Could you check a few things on this model? Use its own coordinates, in mm. A direction names the side the tool comes from. Give positions to 0.01 mm unless a question says otherwise; leave off trailing zeros. Loops run counter-clockwise (first coordinate to the right, second up) from the corner with the lowest first, then second, coordinate; pieces in that order, holes last. Notation, with made-up numbers: M 24,-7.5 L 53,-7.5 A21 ccw 53,3.5 Z; hole C 59.25,-6 d7. An arc over 180 degrees is marked long. Answer in a Markdown table with one row per item. Add a question column.
1. I'm going to push flat-ended pins straight in: pin 1 Ø3 at (x, z) = (84.8, -39.5) entering from -Y; pin 2 Ø3.5 at (y, z) = (1, -13) entering from -X; pin 3 Ø1.5 at (y, z) = (1, -22) entering from +X. Where does each tip first touch, or does it pass through?
2. If we section it at A-A on x = 108: List the corners of the cut face in (y, z) for me, then the cut area to 4 significant figures.
3. If we section it at B-B on z = -8: Count the separate pieces of the cut face and the enclosed holes in it, then the cut area to 3 significant figures.
4. Which directions (+Z, -Z, +X, -X, +Y, -Y) give clear straight access to the entire face, cutting with the end or side of a thin tool? Please do faces 4 (the flat face through (45, 9, -2.9)), 5 (the flat face through (12, 3, -23)), 6 (the flat face through (51.9, 9, -1)), 7 (the flat face through (37, 4, -39)), 8 (the flat face through (120, 4, -23)).
5. If we section it at D-D on z = -22: List the corners of the cut face in (x, y) for me.
6. Thinking about a two-plate mould opening in X: for faces 1 (the cylindrical face through (36.567, 6.958, -39.803)), 2 (the flat face through (108, 3, -23)), 3 (the flat face through (96, 1, -23)), which applies, released by +X, released by -X, zero draft, split by the parting line, or undercut?
7. If we section it at C-C on x = 72.5: List the corners of the cut face in (y, z) for me, then the cut area to 3 significant figures.
8. I need wall thicknesses on line 1 along Z through (x, y) = (108, 3.95); line 2 along X through (y, z) = (4.9, -8); line 3 along Z through (x, y) = (77, 8.75). Which ranges of each line are inside material? Lowest first, please. Write a range as from..to.
Autodesk Inventor part; units mm, degrees
ref_plane "YZ Plane" through (0, 0, 0) normal (1, 0, 0) x (0, 1, 0)
ref_plane "XZ Plane" through (0, 0, 0) normal (0, 1, 0) x (-1, 0, 0)
ref_plane "XY Plane" through (0, 0, 0) normal (0, 0, 1) x (1, 0, 0)
sketch "スケッチ1" plane through (0, 0, 0) normal (0, 1, 0) x (-1, 0, 0)
  line L0 (0, 0) -> (-120, 0)
  line L1 (-120, 0) -> (-120, -47.5)
  line L2 (-120, -47.5) -> (0, -47.5)
  line L3 (0, -47.5) -> (0, 0)
  dimension "d0" = 120
  dimension "d1" = 47.5
extrude "押し出し1" add sketch "スケッチ1" along normal blind 6
ref_plane "作業平面1" through (0, 0, 0) normal (0, 0, 1) x (1, 0, 0)
ref_plane "作業平面2" through (0, 6, 0) normal (0, 1, 0) x (1, 0, 0)
sketch "スケッチ3" plane through (0, 6, 0) normal (0, 1, 0) x (1, 0, 0)
  line L0 (120, 47.5) -> (0, 47.5)
  line L1 (0, 0) -> (120, 0)
  line L2 (30, 47.5) -> (90, 47.5)
  line L3 (90, 47.5) -> (90, 0)
  line L4 (90, 0) -> (30, 0)
  line L5 (30, 0) -> (30, 47.5)
  point P0 (30, 0)
  point P1 (60, 47.5)
  point P2 (60, 47.5)
  point P3 (60, 47.5)
  dimension "d9" = 60
  dimension "d50" = 0
extrude "押し出し3" add sketch "スケッチ3" along normal blind 4
ref_plane "作業平面3" through (0, 10, 0) normal (0, 1, 0) x (1, 0, 0)
sketch "スケッチ4" plane through (0, 10, 0) normal (0, 1, 0) x (1, 0, 0)
  line L0 (38.7, 45.5) -> (81.3, 45.5)
  line L1 (81.3, 45.5) -> (81.3, 2.9)
  line L2 (81.3, 2.9) -> (38.7, 2.9)
  line L3 (38.7, 2.9) -> (38.7, 45.5)
  line L4 (90, 47.5) -> (30, 47.5)
  line L5 (90, 0) -> (90, 47.5)
  point P0 (0, 0)
  point P1 (90, 23.75)
  point P2 (60, 47.5)
  dimension "d14" = 42.6
  dimension "d15" = 42.6
extrude "押し出し4" cut sketch "スケッチ4" against normal blind 2
sketch "スケッチ5" plane through (120, 0, 0) normal (0, 0, 1) x (1, 0, 0)
  line L0 (-30, 10) -> (-90, 10)
  line L1 (-38.7, 8) -> (-81.3, 8)
  line L2 (-68.1, 10) -> (-51.9, 10)
  line L3 (-51.9, 10) -> (-51.9, 8)
  line L4 (-51.9, 8) -> (-68.1, 8)
  line L5 (-68.1, 8) -> (-68.1, 10)
  point P0 (-120, 0)
  dimension "d20" = 16.2
extrude "押し出し5" cut sketch "スケッチ5" against normal blind 3
sketch "スケッチ6" plane through (0, 10, 0) normal (0, 1, 0) x (1, 0, 0)
  line L0 (90, 47.5) -> (30, 47.5)
  line L1 (144, 0) -> (-24, 0)
  line L2 (30, 47.5) -> (30, 0)
  line L3 (90, 0) -> (90, 47.5)
  line L4 (38.7, 2.9) -> (38.7, 45.5)
  point P0 (0, 0)
  point P1 (35.2, 39.5)
  point P2 (35.2, 8)
  point P3 (84.8, 8)
  point P4 (84.8, 39.5)
  dimension "d27" = 8
  dimension "d28" = 8
  dimension "d29" = 8
  dimension "d30" = 8
  dimension "d31" = 5.2
  dimension "d32" = 5.2
  dimension "d33" = 5.2
  dimension "d34" = 5.2
  dimension "d49" = 49.6
  dimension "d75" = 3.5
hole "穴1" at (35.2, 10, -39.5) at (35.2, 10, -8) at (84.8, 10, -8) at (84.8, 10, -39.5) direction (0, -1, 0) diameter 2.8 end through all
sketch "スケッチ7" plane through (0, 0, 0) normal (0, -1, 0) x (1, 0, 0)
  circle A0 centre (35.2, -8) radius 1.4
  circle A1 centre (35.2, -8) radius 3.5
  circle A2 centre (84.8, -8) radius 1.4
  circle A3 centre (84.8, -8) radius 3.5
  circle A4 centre (84.8, -39.5) radius 1.4
  circle A5 centre (84.8, -39.5) radius 3.5
  circle A6 centre (35.2, -39.5) radius 1.4
  circle A7 centre (35.2, -39.5) radius 3.5
  point P0 (0, 0)
  dimension "d42" = 7
  dimension "d43" = 7
  dimension "d44" = 7
  dimension "d45" = 7
extrude "押し出し6" cut sketch "スケッチ7" against normal blind 4 contours A0 | A1 | A3 | A4 | A5 | A6 | A7
ref_plane "作業平面4" through (0, 0, 0) normal (0, -1, 0) x (1, 0, 0)
sketch "スケッチ8" plane through (0, 0, 0) normal (0, -1, 0) x (1, 0, 0)
  line L0 (0, 0) -> (24, 0)
  line L1 (24, 0) -> (24, -47.5)
  line L2 (24, -47.5) -> (0, -47.5)
  line L3 (0, -47.5) -> (0, 0)
  line L4 (120, 0) -> (120, -47.5)
  line L5 (120, 0) -> (96, 0)
  line L6 (96, 0) -> (96, -47.5)
  line L7 (96, -47.5) -> (120, -47.5)
  line L8 (120, -47.5) -> (120, 0)
  dimension "d53" = 24
  dimension "d54" = 47.5
  dimension "d55" = 24
  dimension "d56" = 47.5
extrude "押し出し7" cut sketch "スケッチ8" against normal blind 3
ref_plane "作業平面5" through (0, 3, 0) normal (0, -1, 0) x (1, 0, 0)
sketch "スケッチ9" plane through (0, 3, 0) normal (0, -1, 0) x (1, 0, 0)
  line L0 (0, -47.5) -> (0, 0)
  line L1 (0, 0) -> (24, 0)
  line L2 (24, -47.5) -> (0, -47.5)
  line L3 (120, 0) -> (120, -47.5)
  line L4 (96, 0) -> (120, 0)
  line L5 (120, -47.5) -> (96, -47.5)
  line L6 (24, 0) -> (24, -47.5)
  point P0 (12, -8)
  point P1 (12, -39.5)
  point P2 (108, -8)
  point P3 (108, -39.5)
  point P4 (12, 0)
  dimension "d60" = 12
  dimension "d61" = 8
  dimension "d62" = 8
  dimension "d63" = 12
  dimension "d64" = 12
  dimension "d65" = 12
  dimension "d66" = 8
  dimension "d67" = 8
  dimension "d76" = 12
hole "穴2" at (12, 3, -8) at (12, 3, -39.5) at (108, 3, -8) at (108, 3, -39.5) direction (0, 1, 0) diameter 6 end through all
properties part number "motor_mount1_3D プリント"
Results:
| question | item | result |
|---|---|---|
| 1 | pin 1 | y = 4 |
| 1 | pin 2 | x = 24 |
| 1 | pin 3 | x = 96 |
| 2 | outline | M 3,-47.5 L 6,-47.5 L 6,-42.5 L 3,-42.5 Z; M 3,-36.5 L 6,-36.5 L 6,-11 L 3,-11 Z; M 3,-5 L 6,-5 L 6,0 L 3,0 Z |
| 2 | area | 106.5 mm2 |
| 3 | separate pieces | 5 |
| 3 | enclosed holes | 0 |
| 3 | area | 605 mm2 |
| 4 | face 4 | +Y |
| 4 | face 5 | +Z, -Z, -X, -Y |
| 4 | face 6 | +Z, +Y |
| 4 | face 7 | -Y |
| 4 | face 8 | +Z, -Z, +X, +Y, -Y |
| 5 | outline | M 0,3 L 24,3 L 24,0 L 96,0 L 96,3 L 120,3 L 120,6 L 90,6 L 90,10 L 81.3,10 L 81.3,8 L 38.7,8 L 38.7,10 L 30,10 L 30,6 L 0,6 Z |
| 6 | face 1 | undercut |
| 6 | face 2 | zero draft |
| 6 | face 3 | released by +X |
| 7 | outline | M 0,-47.5 L 10,-47.5 L 10,-45.5 L 8,-45.5 L 8,-2.9 L 10,-2.9 L 10,0 L 0,0 Z |
| 7 | area | 390 mm2 |
| 8 | line 1 | -47.5..-42.5, -36.5..-11, -5..0 |
| 8 | line 2 | 0..9, 15..33.8, 36.6..83.4, 86.2..105, 111..120 |
| 8 | line 3 | -47.5..-45.5, -2.9..0 |
